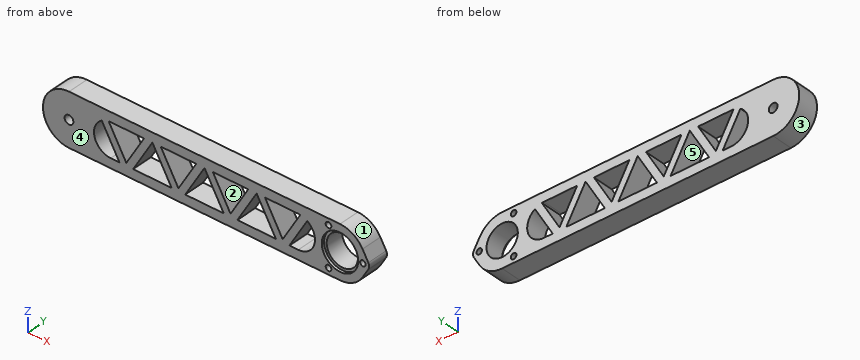
```python
from build123d import *

# Parameters (mm, degrees)
EXTRUDE_1_DEPTH        = 10
EXTRUDE_5_DEPTH        = 10
CUT_EXTRUDE_2_REACH    = 82.606
SKETCH_7_R             = 7.5
SKETCH_8_R             = 8.75
CUT_EXTRUDE_3_DEPTH    = 1.3
CUT_EXTRUDE_4_REACH    = 82.606
SKETCH_9_R             = 1.35
CUT_EXTRUDE_5_REACH    = 82.606
SKETCH_12_R            = 2.1
CUT_EXTRUDE_6_REACH    = 82.606
EXTRUDE_6_DEPTH        = 10
PATTERN_LINEAR_1_DEPTH = 10


# Read off the part's stored shape, not the designer's step: 阵列(线性)1
with BuildPart() as part:
    # 草图1 → 凸台-拉伸1 (new body)
    with BuildSketch(Plane(origin=(0, 0, 0), x_dir=(1, 0, 0), z_dir=(0, 1, 0))):
        with BuildLine():
            Line((-65, 12.5), (65, 12.5))
            ThreePointArc((65, 12.5), (77.5, 0), (65, -12.5))
            Line((65, -12.5), (-65, -12.5))
            ThreePointArc((-65, -12.5), (-77.5, 0), (-65, 12.5))
        make_face()
    extrude(amount=EXTRUDE_1_DEPTH)

    # 草图10 → 凸台-拉伸5 (add)
    with BuildSketch(Plane.XZ):
        with BuildLine():
            Line((75.795454545, -6.301441197), (78.590909091, -1.512345887))
            ThreePointArc((78.590909091, -1.512345887), (79, 0), (78.590909091, 1.512345887))
            Line((78.590909091, 1.512345887), (75.795454545, 6.301441197))
            Line((75.795454545, 6.301441197), (75.795454545, -6.301441197))
        make_face()
    extrude(amount=-EXTRUDE_5_DEPTH)

    # 草图7 → 切除-拉伸2 (cut, up to next)
    with BuildSketch(Plane(origin=(0, 10, 0), x_dir=(1, 0, 0), z_dir=(0, 1, 0)), mode=Mode.PRIVATE) as cut_extrude_2_sk1:
        with Locations(Location((65, 0, 0), (0, 0, 270))):
            Circle(SKETCH_7_R)
    cut_extrude_2_tool1 = extrude(cut_extrude_2_sk1.sketch, amount=-CUT_EXTRUDE_2_REACH, mode=Mode.PRIVATE) & part.part
    add(cut_extrude_2_tool1.solids().sort_by_distance((65, 10, 0))[0], mode=Mode.SUBTRACT)

    # 草图8 → 切除-拉伸3 (cut)
    with BuildSketch(Plane(origin=(0, 0, 0), x_dir=(1, 0, 0), z_dir=(0, 1, 0))):
        with Locations(Location((65, 0, 0), (0, 0, 270))):
            Circle(SKETCH_8_R)
    extrude(amount=CUT_EXTRUDE_3_DEPTH, mode=Mode.SUBTRACT)

    # 草图9 → 切除-拉伸4 (cut, up to next)
    with BuildSketch(Plane.XZ, mode=Mode.PRIVATE) as cut_extrude_4_sk1:
        with Locations(Location((59.5, 9.526279442, 0), (0, 0, 270))):
            Circle(SKETCH_9_R)
    cut_extrude_4_tool1 = extrude(cut_extrude_4_sk1.sketch, amount=-CUT_EXTRUDE_4_REACH, mode=Mode.PRIVATE) & part.part
    # 草图9 → 切除-拉伸4 (cut, up to next)
    with BuildSketch(Plane.XZ, mode=Mode.PRIVATE) as cut_extrude_4_sk2:
        with Locations(Location((76, 0, 0), (0, 0, 270))):
            Circle(SKETCH_9_R)
    cut_extrude_4_tool2 = extrude(cut_extrude_4_sk2.sketch, amount=-CUT_EXTRUDE_4_REACH, mode=Mode.PRIVATE) & part.part
    # 草图9 → 切除-拉伸4 (cut, up to next)
    with BuildSketch(Plane.XZ, mode=Mode.PRIVATE) as cut_extrude_4_sk3:
        with Locations(Location((59.5, -9.526279442, 0), (0, 0, 270))):
            Circle(SKETCH_9_R)
    cut_extrude_4_tool3 = extrude(cut_extrude_4_sk3.sketch, amount=-CUT_EXTRUDE_4_REACH, mode=Mode.PRIVATE) & part.part
    add(cut_extrude_4_tool1.solids().sort_by_distance((59.5, 0, 9.526279))[0], mode=Mode.SUBTRACT)
    add(cut_extrude_4_tool2.solids().sort_by_distance((76, 0, 0))[0], mode=Mode.SUBTRACT)
    add(cut_extrude_4_tool3.solids().sort_by_distance((59.5, 0, -9.526279))[0], mode=Mode.SUBTRACT)

    # 草图12 → 切除-拉伸5 (cut, up to next)
    with BuildSketch(Plane(origin=(0, 10, 0), x_dir=(1, 0, 0), z_dir=(0, 1, 0)), mode=Mode.PRIVATE) as cut_extrude_5_sk1:
        with Locations(Location((-65, 0, 0), (0, 0, 270))):
            Circle(SKETCH_12_R)
    cut_extrude_5_tool1 = extrude(cut_extrude_5_sk1.sketch, amount=-CUT_EXTRUDE_5_REACH, mode=Mode.PRIVATE) & part.part
    add(cut_extrude_5_tool1.solids().sort_by_distance((-65, 10, 0))[0], mode=Mode.SUBTRACT)

    # 草图13 → 切除-拉伸6 (cut, up to next)
    with BuildSketch(Plane(origin=(0, 10, 0), x_dir=(1, 0, 0), z_dir=(0, 1, 0)), mode=Mode.PRIVATE) as cut_extrude_6_sk1:
        with BuildLine():
            Line((-45, 8), (45, 8))
            ThreePointArc((45, 8), (53, 0), (45, -8))
            Line((45, -8), (-45, -8))
            ThreePointArc((-45, -8), (-53, 0), (-45, 8))
        make_face()
    cut_extrude_6_tool1 = extrude(cut_extrude_6_sk1.sketch, amount=-CUT_EXTRUDE_6_REACH, mode=Mode.PRIVATE) & part.part
    add(cut_extrude_6_tool1.solids().sort_by_distance((0, 10, 0))[0], mode=Mode.SUBTRACT)

    # 草图14 → 凸台-拉伸6 (add)
    with BuildSketch(Plane(origin=(0, 10, 0), x_dir=(1, 0, 0), z_dir=(0, 1, 0))):
        Polygon((0, -8), (9.237604307, 8), (13.237604307, 8), (4, -8), align=None)
    extrude_6 = extrude(amount=-EXTRUDE_6_DEPTH)

    # 阵列(线性)1 outline → 阵列(线性)1 (add)
    with BuildSketch(Plane(origin=(0, 0, 0), x_dir=(1, 0, 0), z_dir=(0, 1, 0))):
        Polygon((38.237604307, 8), (34.237604307, 8), (25, -8), (29, -8), align=None)
        Polygon((-11.762395693, 8), (-15.762395693, 8), (-25, -8), (-21, -8), align=None)
        with BuildLine():
            Line((-45.966190603, -7.941440406), (-36.762395693, 8))
            Line((-36.762395693, 8), (-40.762395693, 8))
            Line((-40.762395693, 8), (-49.282491188, -6.757238284))
            ThreePointArc((-49.282491188, -6.757238284), (-47.690306451, -7.534072683), (-45.966190603, -7.941440406))
        make_face()
    pattern_linear_1 = extrude(amount=PATTERN_LINEAR_1_DEPTH)

    # 镜向1: 凸台-拉伸6, 阵列(线性)1 across plane
    add(extrude_6.mirror(Plane(origin=(0, 0, 0), x_dir=(0, 0, 1), z_dir=(1, 0, 0))))
    add(pattern_linear_1.mirror(Plane(origin=(0, 0, 0), x_dir=(0, 0, 1), z_dir=(1, 0, 0))))


solid = part.part
```
The listing builds one solid part. Answer for the finished solid, in the listing's coordinates (mm). Face numbers are marked on the shaded views. A direction names the side the tool comes from. Give positions to 0.01 mm unless a question says otherwise; leave off trailing zeros. Order: outer loops, then holes, each group sorted by start corner. A loop starts at its lowest first (then second) coordinate and runs counter-clockwise, first axis right, second up. Notation, with made-up numbers: (13, 21.25) - (61, 21.25) arc R7 ccw to (61, 29.25) - close; hole circle Ø8 at (24.25, 14). An arc over 180 degrees is marked (long way). Use one line per item in the form item = value. Start each with the question number.
(1) For the marked faces 1 and 2, determine the directions among +Z, -Z, +X, -X, +Y, -Y from which every point of the face is accessible in a straight line to the end or side of a thin tool.
(2) A cutting plane is placed at A-A, the plane x = 63. Write down the section's boundary in (y, z), then the cut area to 3 significant figures.
(3) The mould has two halves that part along X. Classify the marked faces 3, 4 and 5: released by +X, released by -X, zero draft, split by the parting line, or undercut.
(4) Flat-ended cylindrical pins translate along their axes: pin 1 Ø4 at (y, z) = (9, -5) entering from +X; pin 2 Ø6.5 at (x, z) = (-65, 0) entering from -Y; pin 3 Ø5 at (y, z) = (5, 8) entering from +X; pin 4 Ø5 at (y, z) = (2.5, 5) entering from +X. Find the tip coordinate at first contact, or state that the pin passes through.
(5) A cutting plane is placed at B-B, the plane y = 4.5. State how many separate pieces and enclosed holes the cut face has, then the cut area to 3 significant figures.
(6) Consider line 1 (Z direction, x = -18, y = 6.5); line 2 (Z direction, x = -31.5, y = 5.5); line 3 (Z direction, x = -14.5, y = 7.5). Determine where each line is inside the solid, lowest interval first. Write a range as from..to.
Ans:
q1.face_1 = +Z, +X, +Y, -Y
q1.face_2 = +Y, -Y
q2.outline = (0, -12.5) - (10, -12.5) - (10, -7.23) - (1.3, -7.23) - (1.3, -8.52) - (0, -8.52) - close; (0, 8.52) - (1.3, 8.52) - (1.3, 7.23) - (10, 7.23) - (10, 12.5) - (0, 12.5) - close
q2.area = 102 mm^2
q3.face_3 = released by -X
q3.face_4 = zero draft
q3.face_5 = undercut
q4.pin_1 = 77.72
q4.pin_2 = 0
q4.pin_3 = 76.26
q4.pin_4 = 78.01
q5.separate_pieces = 1
q5.enclosed_holes = 14
q5.area = 2,400 mm^2
q6.line_1 = -12.5..-8, -4.12..2.8, 8..12.5
q6.line_2 = -12.5..-8, -3.26..3.67, 8..12.5
q6.line_3 = -12.5..-3.26, 8..12.5
